Read the model definition and answer for the solid it produces. Units are mm, in the model's axes. A direction names the side the tool comes from. Give positions to 0.01 mm unless a question says otherwise; leave off trailing zeros. Loops run counter-clockwise (first coordinate to the right, second up) from the corner with the lowest first, then second, coordinate; pieces in that order, holes last. Notation, with made-up numbers: (40, -5) - (53, -5) arc R24 ccw to (53, 30) - close; hole circle Ø1 at (-36, -30). An arc over 180 degrees is marked (long way). Put each result on its own line as item: value. Start each with the question number.
1. Given pin 1 Ø20.5 at (x, y) = (3, 83.5) entering from -Z; pin 2 Ø6 at (y, z) = (-39, 39) entering from -X; pin 3 Ø5 at (y, z) = (61.5, 20.5) entering from -X, each flat-ended and moving along its own axis, determine where each tip first touches the part or whether it passes through.
2. A cutting plane is placed at A-A, the plane z = 12. Count the separate pieces of the cut face and the enclosed holes in it, plus the area to 3 significant figures.
3. A cutting plane is placed at C-C, the plane y = 26. Determine the outline of the cut face in (x, z), plus the area to 3 significant figures.
4. Consider L1, parallel to Y at x = 0, z = 29; L2, parallel to Y at x = -17, z = 8.5; L3, parallel to X at y = -77, z = 16.5. Determine where each line is inside the solid, lowest interval first. Write a range as from..to.
5. For a pull along X with two mould halves and no side action, classify faces 4 (the flat face through (-70, 14, 0)), 5 (the flat face through (17, 66.5, 9.9)), 6 (the cylindrical face through (40.057, -40.255, 39.528)) as released by +X, released by -X, zero draft, split by the parting line, or undercut.
6. A cutting plane is placed at D-D, the plane y = -81.5. Determine the outline of the cut face in (x, z).
7. For faces 1 (the flat face through (48.86, 34.72, 34.06)), 2 (the flat face through (0, 81, 20)), 3 (the flat face through (-81, 0, 20)), determine the directions among +Z, -Z, +X, -X, +Y, -Y from which every point of the face is accessible in a straight line to the end or side of a thin tool.
8. A cutting plane is placed at B-B, the plane z = 27.5. Determine the outline of the cut face in (x, y), plus the area to 3 significant figures.
```python
from build123d import *

# Parameters (mm, degrees)
SALIENTE_EXTRUIR1_DEPTH   = 20
SALIENTE_EXTRUIR1_2_DEPTH = 20
SALIENTE_EXTRUIR1_3_DEPTH = 20
SALIENTE_EXTRUIR1_4_DEPTH = 20
SALIENTE_EXTRUIR1_5_DEPTH = 20
SALIENTE_EXTRUIR1_6_DEPTH = 20
SALIENTE_EXTRUIR1_7_DEPTH = 20
SALIENTE_EXTRUIR1_8_DEPTH = 20
SALIENTE_EXTRUIR2_DEPTH   = 10
CROQUIS7_R                = 3
CORTAR_EXTRUIR2_DEPTH     = 80
CROQUIS8_R                = 3
CORTAR_EXTRUIR3_DEPTH     = 10
SIMETR_A4_COPY_1_SKETCH_R = 3
SIMETR_A4_COPY_1_DEPTH    = 80
SIMETR_A4_COPY_2_SKETCH_R = 3
SIMETR_A4_COPY_2_DEPTH    = 10
SALIENTE_EXTRUIR3_DEPTH   = 15
CROQUIS11_R               = 3
CORTAR_EXTRUIR4_DEPTH     = 150.913308282
CROQUIS13_R               = 3
CORTAR_EXTRUIR5_DEPTH     = 150.913308282


with BuildPart() as part:
    # Croquis1 → Saliente-Extruir1 (new body)
    with BuildSketch(Plane.XY):
        Polygon((-71.77133829, 22.273863607), (-61.164736573, 11.66726189), (-68.235804385, 4.596194078), (-78.842406102, 15.202795796), align=None)
    extrude(amount=SALIENTE_EXTRUIR1_DEPTH)



with BuildPart() as body_2:
    # Croquis1 → Saliente-Extruir1 2 (new body)
    with BuildSketch(Plane.XY):
        Polygon((-11.66726189, 61.164736573), (-4.596194078, 68.235804385), (-15.202795796, 78.842406102), (-22.273863607, 71.77133829), align=None)
    extrude(amount=SALIENTE_EXTRUIR1_2_DEPTH)


with BuildPart() as body_3:
    # Croquis1 → Saliente-Extruir1 3 (new body)
    with BuildSketch(Plane.XY):
        Polygon((22.273863607, 71.77133829), (11.66726189, 61.164736573), (4.596194078, 68.235804385), (15.202795796, 78.842406102), align=None)
    extrude(amount=SALIENTE_EXTRUIR1_3_DEPTH)


with BuildPart() as body_4:
    # Croquis1 → Saliente-Extruir1 4 (new body)
    with BuildSketch(Plane.XY):
        Polygon((61.164736573, 11.66726189), (68.235804385, 4.596194078), (78.842406102, 15.202795796), (71.77133829, 22.273863607), align=None)
    extrude(amount=SALIENTE_EXTRUIR1_4_DEPTH)


with BuildPart() as body_5:
    # Croquis1 → Saliente-Extruir1 5 (new body)
    with BuildSketch(Plane.XY):
        Polygon((71.77133829, -22.273863607), (61.164736573, -11.66726189), (68.235804385, -4.596194078), (78.842406102, -15.202795796), align=None)
    extrude(amount=SALIENTE_EXTRUIR1_5_DEPTH)


with BuildPart() as body_6:
    # Croquis1 → Saliente-Extruir1 6 (new body)
    with BuildSketch(Plane.XY):
        Polygon((11.66726189, -61.164736573), (4.596194078, -68.235804385), (15.202795796, -78.842406102), (22.273863607, -71.77133829), align=None)
    extrude(amount=SALIENTE_EXTRUIR1_6_DEPTH)


with BuildPart() as body_7:
    # Croquis1 → Saliente-Extruir1 7 (new body)
    with BuildSketch(Plane.XY):
        Polygon((-22.273863607, -71.77133829), (-11.66726189, -61.164736573), (-4.596194078, -68.235804385), (-15.202795796, -78.842406102), align=None)
    extrude(amount=SALIENTE_EXTRUIR1_7_DEPTH)


with BuildPart() as body_8:
    # Croquis1 → Saliente-Extruir1 8 (new body)
    with BuildSketch(Plane.XY):
        Polygon((-61.164736573, -11.66726189), (-68.235804385, -4.596194078), (-78.842406102, -15.202795796), (-71.77133829, -22.273863607), align=None)
    extrude(amount=SALIENTE_EXTRUIR1_8_DEPTH)


with BuildPart() as part_1:
    add(part.part)

    add(body_2.part)  # Saliente-Extruir2 merges body 2

    add(body_3.part)  # Saliente-Extruir2 merges body 3

    add(body_4.part)  # Saliente-Extruir2 merges body 4

    add(body_5.part)  # Saliente-Extruir2 merges body 5

    add(body_6.part)  # Saliente-Extruir2 merges body 6

    add(body_7.part)  # Saliente-Extruir2 merges body 7

    add(body_8.part)  # Saliente-Extruir2 merges body 8
    # Croquis2 → Saliente-Extruir2 (add)
    with BuildSketch(Plane.XY.offset(20)):
        Polygon((0, 94.045201898), (94.045201898, 0), (0, -94.045201898), (-94.045201898, 0), align=None)
        Polygon((0, 72.831998462), (72.831998462, 0), (0, -72.831998462), (-72.831998462, 0), align=None, mode=Mode.SUBTRACT)
    extrude(amount=SALIENTE_EXTRUIR2_DEPTH)

    # Croquis7 → Cortar-Extruir2 (cut)
    with BuildSketch(Plane(origin=(31.819805153, 31.819805153, 0), x_dir=(0, 0, -1), z_dir=(0.7071067811865476, 0.7071067811865476, 0))):
        with Locations(Location((-5, -59, 0), (0, 0, 90))):
            Circle(CROQUIS7_R)
    cortar_extruir2 = extrude(amount=-CORTAR_EXTRUIR2_DEPTH, mode=Mode.SUBTRACT)

    # Croquis8 → Cortar-Extruir3 (cut)
    with BuildSketch(Plane(origin=(31.819805153, -31.819805153, 0), x_dir=(0, 0, -1), z_dir=(0.7071067811865481, -0.707106781186547, 0))):
        with Locations(Location((-5, 59, 0), (0, 0, 90))):
            Circle(CROQUIS8_R)
    cortar_extruir3 = extrude(amount=-CORTAR_EXTRUIR3_DEPTH, mode=Mode.SUBTRACT)

    # Simetría3: Cortar-Extruir2, Cortar-Extruir3 across plane
    add(cortar_extruir2.mirror(Plane(origin=(0, 0, 0), x_dir=(0, 0, 1), z_dir=(0.7071067811865481, -0.707106781186547, 0))), mode=Mode.SUBTRACT)
    add(cortar_extruir3.mirror(Plane(origin=(0, 0, 0), x_dir=(0, 0, 1), z_dir=(0.7071067811865481, -0.707106781186547, 0))), mode=Mode.SUBTRACT)

    # Simetría4: Cortar-Extruir2, Cortar-Extruir3 across plane
    add(cortar_extruir2.mirror(Plane(origin=(0, 0, 0), x_dir=(0, 0, 1), z_dir=(-0.7071067811865477, -0.7071067811865475, 0))), mode=Mode.SUBTRACT)
    add(cortar_extruir3.mirror(Plane(origin=(0, 0, 0), x_dir=(0, 0, 1), z_dir=(-0.7071067811865477, -0.7071067811865475, 0))), mode=Mode.SUBTRACT)

    # Simetría4 copy 1 sketch → Simetría4 copy 1 (cut)
    with BuildSketch(Plane(origin=(-31.819805153, -31.819805153, 0), x_dir=(0, 0, -1), z_dir=(-0.7071067811865492, -0.7071067811865465, 0))):
        with Locations(Location((-5, -59, 0), (0, 0, 90))):
            Circle(SIMETR_A4_COPY_1_SKETCH_R)
    extrude(amount=-SIMETR_A4_COPY_1_DEPTH, mode=Mode.SUBTRACT)

    # Simetría4 copy 2 sketch → Simetría4 copy 2 (cut)
    with BuildSketch(Plane(origin=(-31.819805153, 31.819805153, 0), x_dir=(0, 0, -1), z_dir=(-0.7071067811865471, 0.7071067811865488, 0))):
        with Locations(Location((-5, 59, 0), (0, 0, 90))):
            Circle(SIMETR_A4_COPY_2_SKETCH_R)
    extrude(amount=-SIMETR_A4_COPY_2_DEPTH, mode=Mode.SUBTRACT)

    # Croquis10 → Saliente-Extruir3 (add)
    with BuildSketch(Plane.XY.offset(30)):
        Polygon((29.344931419, 43.487067043), (39.951533137, 54.093668761), (54.093668761, 39.951533137), (43.487067043, 29.344931419), align=None)
        Polygon((43.487067043, -29.344931419), (54.093668761, -39.951533137), (39.951533137, -54.093668761), (29.344931419, -43.487067043), align=None)
        Polygon((-29.344931419, -43.487067043), (-39.951533137, -54.093668761), (-54.093668761, -39.951533137), (-43.487067043, -29.344931419), align=None)
        Polygon((-43.487067043, 29.344931419), (-54.093668761, 39.951533137), (-39.951533137, 54.093668761), (-29.344931419, 43.487067043), align=None)
    extrude(amount=SALIENTE_EXTRUIR3_DEPTH)

    # Croquis11 → Cortar-Extruir4 (cut, through all)
    with BuildSketch(Plane(origin=(7.071067812, -7.071067812, 0), x_dir=(0, 0, -1), z_dir=(0.7071067811865481, -0.707106781186547, 0))):
        with Locations(Location((-37.5, 59, 0), (0, 0, 90))):
            Circle(CROQUIS11_R)
        with Locations(Location((-37.5, -59, 0), (0, 0, 90))):
            Circle(CROQUIS11_R)
    extrude(amount=-CORTAR_EXTRUIR4_DEPTH, mode=Mode.SUBTRACT)

    # Croquis13 → Cortar-Extruir5 (cut, through all)
    with BuildSketch(Plane(origin=(-7.071067812, -7.071067812, 0), x_dir=(0, 0, 1), z_dir=(-0.707106781186549, -0.707106781186546, 0))):
        with Locations(Location((37.5, -59, 0), (0, 0, 270))):
            Circle(CROQUIS13_R)
        with Locations(Location((37.5, 59, 0), (0, 0, 270))):
            Circle(CROQUIS13_R)
    extrude(amount=-CORTAR_EXTRUIR5_DEPTH, mode=Mode.SUBTRACT)


solid = part_1.part
```
Return value:
1. pin 1: stops at z = 20
1. pin 2: stops at x = -54.09
1. pin 3: stops at x = -35.05
2. separate pieces: 8
2. enclosed holes: 0
2. area: 1,200 mm2
3. outline: (-68.05, 20) - (-46.83, 20) - (-46.83, 30) - (-68.05, 30) - close; (46.83, 20) - (68.05, 20) - (68.05, 30) - (46.83, 30) - close
3. area: 424 mm2
4. L1: y = -94.05..-72.83, 72.83..94.05
4. L2: y = -77.05..-66.5, 66.5..77.05
4. L3: x = -17.05..-13.36, 13.36..17.05
5. face 4: zero draft
5. face 5: released by +X
5. face 6: undercut
6. outline: (-12.55, 20) - (12.55, 20) - (12.55, 30) - (-12.55, 30) - close
7. face 1: +Z, +X
7. face 2: -Z, +Y
7. face 3: -Z, -X
8. outline: (-94.05, 0) - (0, -94.05) - (94.05, 0) - (0, 94.05) - close; hole (-72.83, 0) - (0, -72.83) - (72.83, 0) - (0, 72.83) - close
8. area: 7,080 mm2
